Check sheet for the drawn part. Datum: minimum x, y, z corner. Units: mm. Round coordinates to 2 decimals unless told otherwise and drop trailing zeros. Order: outer loops, then holes, each group sorted by start corner. A loop starts at its lowest first (then second) coordinate and runs counter-clockwise, first axis right, second up. Notation, with made-up numbers: M -1,73.25 L 52,73.25 A24 ccw 52,98.25 Z; hole C 76.25,77 d5. An arc over 180 degrees is marked long. Answer as a JSON object with one key per item and string values. Group by question number.
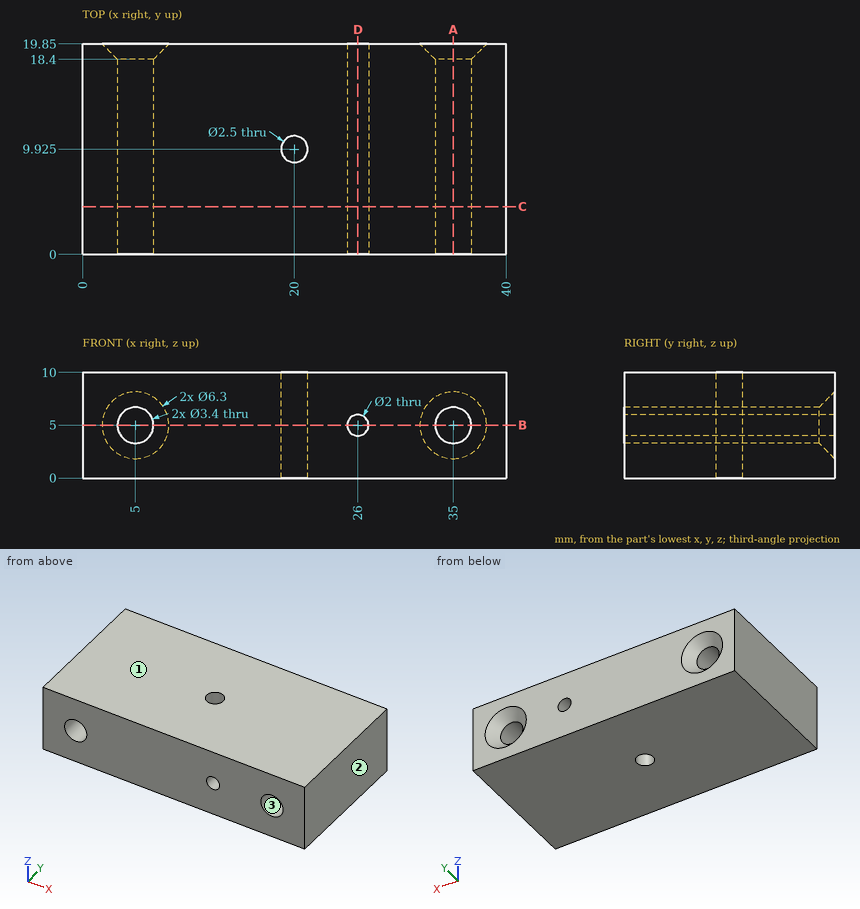
1) Sectioned sample at D-D (x = 26). Record the boundary of the cut face in (y, z).
2) Sectioned sample at C-C (y = 4.5). Record the boundary of the cut face in (x, z), then the cut area to 3 significant figures.
3) Sectioned sample at B-B (z = 5). Record the boundary of the cut face in (x, y) (3 decimals), then the cut area to 3 significant figures.
4) Sectioned sample at A-A (x = 35). Record the boundary of the cut face in (y, z), then the cut area to 3 significant figures.
5) Release check for a two-part mould opening along X. For the marked faces 1, 2 and 3 record: +X half, -X half, draft (parallel to the pull), parting line (faces both ways), or undercut.
6) Thickness scan on line 1 along X through (y, z) = (8, 5); line 2 along X through (y, z) = (10.5, 5); line 3 along X through (y, z) = (14, 4.25). Record the ranges inside material, lowest first. Write a range as [from, to].
Final values:
{
 "1": {"outline": "M 0,0 L 19.85,0 L 19.85,4 L 0,4 Z; M 0,6 L 19.85,6 L 19.85,10 L 0,10 Z"},
 "2": {"outline": "M 0,0 L 40,0 L 40,10 L 0,10 Z; hole C 5,5 d3.4; hole C 26,5 d2; hole C 35,5 d3.4", "area": "379 mm^2"},
 "3": {"outline": "M 0,0 L 3.3,0 L 3.3,18.4 L 1.85,19.85 L 0,19.85 Z; M 6.7,0 L 25,0 L 25,19.85 L 8.15,19.85 L 6.7,18.4 Z; M 27,0 L 33.3,0 L 33.3,18.4 L 31.85,19.85 L 27,19.85 Z; M 36.7,0 L 40,0 L 40,19.85 L 38.15,19.85 L 36.7,18.4 Z; hole C 20,9.925 d2.5", "area": "610 mm^2"},
 "4": {"outline": "M 0,0 L 19.85,0 L 19.85,1.85 L 18.4,3.3 L 0,3.3 Z; M 0,6.7 L 18.4,6.7 L 19.85,8.15 L 19.85,10 L 0,10 Z", "area": "129 mm^2"},
 "5": {"face 1": "draft", "face 2": "+X half", "face 3": "undercut"},
 "6": {"line 1": "x = [0, 3.3], [6.7, 25], [27, 33.3], [36.7, 40]", "line 2": "x = [0, 3.3], [6.7, 18.89], [21.11, 25], [27, 33.3], [36.7, 40]", "line 3": "x = [0, 3.47], [6.53, 25.34], [26.66, 33.47], [36.53, 40]"}
}
